Could you check a few things on this model? Use its own coordinates, in mm. A direction names the side the tool comes from. Give positions to 0.01 mm unless a question says otherwise; leave off trailing zeros. Write each loop counter-clockwise with the first axis right and the second up, starting at its lowest first coordinate (ties: lowest second). Pieces come first, ordered by that corner, then holes. Notation, with made-up numbers: M 36.25,-33 L 48.25,-33 A9 cw 48.25,-25 Z; hole C 17,10.25 d3. An arc over 180 degrees is marked long. Answer as CSV lines item,"result". Start each with the question number.
from build123d import *

# Parameters (mm, degrees)
F3_R          = 2.85
F3_R_2        = 1.5
F4_DEPTH      = 2
F5_R          = 1.5
F6_DEPTH      = 1.5
F6_DEPTH_BACK = 2
F7_SIZE       = 1.49999
F8_T1_DEPTH   = 2
F8_T6_DEPTH   = 5.7994185071
F8_T12_DEPTH  = 5.7994185071


# Not quite as in the source:
# - a fillet or chamfer that OpenCascade refuses, or shapes differently, is made with other operations: its cross-section is extruded or revolved along the edge and cut away or added
# - a fillet or chamfer is up to 0.001 mm smaller than in the source, because OpenCascade refuses the exact size


with BuildPart() as f4:
    # F3 (on Top) → F4 (new body)
    with BuildSketch(Plane.XY):
        with BuildLine():
            ThreePointArc((-19.2101191839, 28.2786664177), (-27.4339393789, 26.1039339801), (-21.8109953554, 19.7208954965))
            Line((-21.8109953554, 19.7208954965), (-17.5, 15.6341847014))
            Line((-17.5, 15.6341847014), (-17.5, -19.8340624222))
            Line((-17.5, -19.8340624222), (-18.9980046584, -21.2348967768))
            ThreePointArc((-18.9980046584, -21.2348967768), (-27.6471933185, -24.4824919767), (-19.2348967768, -28.3019953416))
            Line((-19.2348967768, -28.3019953416), (-14.2924483884, -23.6801462309))
            ThreePointArc((-14.2924483884, -23.6801462309), (-13.7066532067, -22.8494176119), (-13.5, -21.8541485601))
            Line((-13.5, -21.8541485601), (-13.5, 21.1458514399))
            ThreePointArc((-13.5, 21.1458514399), (-13.8252470415, 22.7257852025), (-14.7480953471, 24.0487845741))
            Line((-14.7480953471, 24.0487845741), (-19.2101191839, 28.2786664177))
        make_face()
        with Locations((-22.65, -24.65)):
            Circle(F3_R, mode=Mode.SUBTRACT)
        with Locations((-16, -21.8541485601)):
            Circle(F3_R_2, mode=Mode.SUBTRACT)
        with Locations((-22.65, 24.65)):
            Circle(F3_R, mode=Mode.SUBTRACT)
        with Locations((-17.5, 21.1458514399)):
            Circle(F3_R_2, mode=Mode.SUBTRACT)
    extrude(amount=F4_DEPTH)

    # F5 (on face) → F6 (join, two sides)
    with BuildSketch(Plane.XY.offset(2)) as f6_sk:
        with BuildLine():
            ThreePointArc((-18.9973102923, 21.2356394597), (-20.2798856869, 20.2474373209), (-21.8109953554, 19.7208954965))
            Line((-21.8109953554, 19.7208954965), (-17.5, 15.6341847014))
            Line((-17.5, 15.6341847014), (-13.5, 15.6341847014))
            Line((-13.5, 15.6341847014), (-13.5, 21.1458514399))
            ThreePointArc((-13.5, 21.1458514399), (-13.8252470415, 22.7257852025), (-14.7480953471, 24.0487845741))
            Line((-14.7480953471, 24.0487845741), (-19.2101191839, 28.2786664177))
            ThreePointArc((-19.2101191839, 28.2786664177), (-17.7347965939, 25.5669380986), (-18.1331588264, 22.5056712444))
            ThreePointArc((-18.1331588264, 22.5056712444), (-16.6936930608, 22.410710768), (-16, 21.1458514399))
            ThreePointArc((-16, 21.1458514399), (-17.5449141487, 19.6465240176), (-18.9973102923, 21.2356394597))
        make_face()
        with BuildLine():
            Line((-13.5, -16.9443202766), (-17.5, -16.9443202766))
            Line((-17.5, -16.9443202766), (-17.5, -19.8340624222))
            Line((-17.5, -19.8340624222), (-18.9980046584, -21.2348967768))
            ThreePointArc((-18.9980046584, -21.2348967768), (-18.9888758035, -21.2446850928), (-18.9797731837, -21.2544978108))
            ThreePointArc((-18.9797731837, -21.2544978108), (-17.6532729909, -24.8308844832), (-19.2348967768, -28.3019953416))
            Line((-19.2348967768, -28.3019953416), (-14.2924483884, -23.6801462309))
            ThreePointArc((-14.2924483884, -23.6801462309), (-13.7066532067, -22.8494176119), (-13.5, -21.8541485601))
            Line((-13.5, -21.8541485601), (-13.5, -16.9443202766))
        make_face()
        with Locations((-16, -21.8541485601)):
            Circle(F5_R, mode=Mode.SUBTRACT)
        with BuildLine():
            Line((-17.5, -19.8340624222), (-17.5, -16.9443202766))
            ThreePointArc((-17.5, -16.9443202766), (-18.6859920066, -19.3337501249), (-21.30625, -19.8339501729))
            ThreePointArc((-21.30625, -19.8339501729), (-20.0557697237, -20.3756615396), (-18.9980046584, -21.2348967768))
            Line((-18.9980046584, -21.2348967768), (-17.5, -19.8340624222))
        make_face()
    extrude(amount=F6_DEPTH)
    extrude(f6_sk.sketch, amount=-F6_DEPTH_BACK)

    # F7 (size 1.5 in the source; OpenCascade refuses exactly that, so slightly less here)
    f7_edges = [f4.edges().sort_by_distance(p)[0] for p in [
        (-15.5, -16.94432, 2),
        (-15.5, 15.634185, 2),
    ]]
    chamfer(f7_edges, length=F7_SIZE)

    # F8: fillet of radius 4 on 2 edges, made by hand

    # F8_s2 → F8_t1 (join)
    with BuildSketch(Plane.XY):
        with BuildLine():
            ThreePointArc((-17.5, 13.9144132985), (-17.8252470415, 15.4943470611), (-18.7480953471, 16.8173464327))
            Line((-18.7480953471, 16.8173464327), (-17.5, 15.6341847014))
            Line((-17.5, 15.6341847014), (-17.5, 13.9144132985))
        make_face()
        with BuildLine():
            ThreePointArc((-23.0447031853, 19.6656034071), (-21.7335895232, 19.3322992897), (-20.6085610806, 18.5810192669))
            Line((-20.6085610806, 18.5810192669), (-21.8109953554, 19.7208954965))
            ThreePointArc((-21.8109953554, 19.7208954965), (-22.4261356427, 19.6550140391), (-23.0447031853, 19.6656034071))
        make_face()
    extrude(amount=F8_T1_DEPTH)


with BuildPart() as f8_tool4:
    # F8_s5 → F8_t6 (new body)
    with BuildSketch(Plane.XY.offset(2)):
        with BuildLine():
            ThreePointArc((-17.5, 13.9144132985), (-17.8252470415, 15.4943470611), (-18.7480953471, 16.8173464327))
            Line((-18.7480953471, 16.8173464327), (-17.5, 15.6341847014))
            Line((-17.5, 15.6341847014), (-17.5, 13.9144132985))
        make_face()
    extrude(amount=F8_T6_DEPTH)

    split(bisect_by=Plane(origin=(0, 6.0670973507, -6.0670973507), x_dir=(1, 0, 0), z_dir=(0, 0.7071067812, -0.7071067812)), keep=Keep.TOP)

    split(bisect_by=Plane.XY.offset(3.5), keep=Keep.BOTTOM)


with BuildPart() as f4_1:
    add(f4.part)

    # F8_t3: union F8_tool4
    add(f8_tool4.part)


with BuildPart() as f8_tool10:
    # F8_s11 → F8_t12 (new body)
    with BuildSketch(Plane.XY.offset(2)):
        with BuildLine():
            ThreePointArc((-17.5, 13.9144132985), (-17.8252470415, 15.4943470611), (-18.7480953471, 16.8173464327))
            Line((-18.7480953471, 16.8173464327), (-17.5, 15.6341847014))
            Line((-17.5, 15.6341847014), (-17.5, 13.9144132985))
        make_face()
    extrude(amount=F8_T12_DEPTH)

    split(bisect_by=Plane.XZ.offset(-15.6341847014), keep=Keep.BOTTOM)

    split(bisect_by=Plane.XY.offset(3.5), keep=Keep.BOTTOM)


with BuildPart() as f4_2:
    add(f4_1.part)

    # F8_t9: union F8_tool10
    add(f8_tool10.part)


solid = f4_2.part
1. Imagine slicing it at A-A, the plane z = 2.95. State how many separate pieces and enclosed holes the cut face has, plus the area to 3 significant figures.
2. Will these pins go through, and if not, where does the flat tip stop? P1, Ø3, axis at x = -15, y = 4.5, coming from the +Z side; P2, Ø1, axis at y = 2.5, z = 2, coming from the -X side; P3, Ø1, axis at x = -23.5, z = 1.5, coming from the +Y side.
3. On a 3-axis mill with a long thin cutter (end or side, diameter ignored), from which of +Z, -Z, +X, -X, +Y, -Y can I reach the whole of each face in a straight line? I mean faces 1 (the flat face through (-17.5, -1, 1)), 2 (the flat face through (-15.472, -16.184, 2.739)), 3 (the cylindrical face through (-18.655, -19.31, 1.774)). Say none if no direction works.
4. Imagine slicing it at B-B, the plane y = -24.65. Please give me the cut outline in (x, z).
5. Thinking about a two-plate mould opening in Y: for faces 4 (the flat face through (-15, 0, 2)), 5 (the flat face through (-16.798, -26.023, 1.726)), 6 (the flat face through (-17, -20, 3.5)), which applies, pulls with the +Y half, pulls with the -Y half, needs draft (parallel to the pull), parting line crosses it, or undercut?
6. Imagine slicing it at C-C, the plane y = 10.5. Please give me the cut outline in (x, z).
7. Please list where these lines run through material, in increasing order: line 1 (Y direction, x = -24.5, z = 0.75); line 2 (Y direction, x = -22.65, z = 1.65); line 3 (Z direction, x = -15, y = 3.5).
Solutions:
1,separate pieces,"2"
1,enclosed holes,"1"
1,area,"81.6 mm²"
2,P1,"z = 2"
2,P2,"x = -17.5"
2,P3,"y = 29.64"
3,face 1,"+Z, -Z, -X"
3,face 2,"+Z, +X, -X"
3,face 3,"+Z, -Z"
4,outline,"M -27.65,0 L -25.5,0 L -25.5,2 L -27.65,2 Z; M -19.8,0 L -15.33,0 L -15.33,3.5 L -17.65,3.5 L -17.65,2 L -19.8,2 Z"
5,face 4,"undercut"
5,face 5,"pulls with the -Y half"
5,face 6,"needs draft"
6,outline,"M -17.5,0 L -13.5,0 L -13.5,2 L -17.5,2 Z"
7,line 1,"-29.3 to -26.82, -22.48 to -20, 20 to 22.48, 26.82 to 29.3"
7,line 2,"-29.65 to -27.5, -21.8 to -19.65, 19.61 to 21.8, 27.5 to 29.65"
7,line 3,"0 to 2"
